from build123d import *
from OCP.BRepFilletAPI import BRepFilletAPI_MakeChamfer

# Parameters (mm, degrees)
BOSS_EXTRUDE1_DEPTH = 9
CUT_EXTRUDE1_REACH  = 32.118
SKETCH2_R           = 6.5
CUT_EXTRUDE2_DEPTH  = 18
CUT_EXTRUDE3_REACH  = 30.95
SKETCH4_R           = 3.7499999999999996
CUT_EXTRUDE4_DEPTH  = 10
FILLET1_R           = 2
CHAMFER1_SIZE       = 2
CHAMFER1_SIZE2      = 0.8842438837908889
CHAMFER1_SIZE2_2    = 0.8842438837908887


with BuildPart() as part:
    # Sketch1 → Boss-Extrude1 (new, symmetric)
    with BuildSketch(Plane.XY):
        Polygon((-25.633576548445145, 1e-17), (-11.506423451554879, 4e-17), (-8, 10), (0, 9.999999999999993), (8, 9.999999999999993), (11.506423451554879, 4e-17), (25.633576548445145, 4e-17), (25.63357654844514, 3.000000000000001), (13.633576548445141, 3), (10.12715309689026, 13.000000000000002), (0, 12.999999999999995), (-10.127153096890261, 13.000000000000002), (-13.633576548445141, 3), (-25.633576548445145, 3), align=None)
    extrude(amount=BOSS_EXTRUDE1_DEPTH, both=True)

    # Sketch2 → Cut-Extrude1 (cut, up to next)
    with BuildSketch(Plane(origin=(8.91e-15, 12.999999999999995, 0), x_dir=(1, -7.1e-16, 0), z_dir=(7.1e-16, 1, 0)), mode=Mode.PRIVATE) as cut_extrude1_sk1:
        with Locations(Location((0, 0, 0), (0, 0, 180))):
            Circle(SKETCH2_R)
    cut_extrude1_tool1 = extrude(cut_extrude1_sk1.sketch, amount=-CUT_EXTRUDE1_REACH, mode=Mode.PRIVATE) & part.part
    add(cut_extrude1_tool1.solids().sort_by_distance((0, 13, 0))[0], mode=Mode.SUBTRACT)

    # Sketch3 → Cut-Extrude2 (cut)
    with BuildSketch(Plane(origin=(8.91e-15, 12.999999999999995, 0), x_dir=(1, -7.1e-16, 0), z_dir=(7.1e-16, 1, 0))):
        Polygon((-10.12715309689027, 9), (-25.63357654844515, 4), (-25.63357654844515, 9), align=None)
        Polygon((-10.12715309689025, -9), (-25.63357654844515, -4), (-25.63357654844515, -9), align=None)
        Polygon((25.63357654844515, 9), (10.12715309689025, 9), (25.63357654844515, 4), align=None)
        Polygon((25.63357654844515, -4), (25.63357654844515, -9), (10.12715309689025, -9), align=None)
    extrude(amount=-CUT_EXTRUDE2_DEPTH, mode=Mode.SUBTRACT)

    # Sketch4 → Cut-Extrude3 (cut, up to next)
    with BuildSketch(Plane(origin=(0, 3, 0), x_dir=(1, 0, 0), z_dir=(0, 1, 0)), mode=Mode.PRIVATE) as cut_extrude3_sk1:
        with Locations(Location((-19.633576548445145, -2.4e-15, 0), (0, 0, 270))):
            Circle(SKETCH4_R)
    cut_extrude3_tool1 = extrude(cut_extrude3_sk1.sketch, amount=-CUT_EXTRUDE3_REACH, mode=Mode.PRIVATE) & part.part
    # Sketch4 → Cut-Extrude3 (cut, up to next)
    with BuildSketch(Plane(origin=(0, 3, 0), x_dir=(1, 0, 0), z_dir=(0, 1, 0)), mode=Mode.PRIVATE) as cut_extrude3_sk2:
        with Locations(Location((19.63357654844515, 2.4e-15, 0), (0, 0, 270))):
            Circle(SKETCH4_R)
    cut_extrude3_tool2 = extrude(cut_extrude3_sk2.sketch, amount=-CUT_EXTRUDE3_REACH, mode=Mode.PRIVATE) & part.part
    add(cut_extrude3_tool1.solids().sort_by_distance((-19.633577, 3, 0))[0], mode=Mode.SUBTRACT)
    add(cut_extrude3_tool2.solids().sort_by_distance((19.633577, 3, 0))[0], mode=Mode.SUBTRACT)

    # Sketch5 → Cut-Extrude4 (cut, symmetric)
    with BuildSketch(Plane.XY):
        Polygon((13.633576548445141, 3), (14.247200652467244, 1.2500000000000009), (25.63357654844515, 1.2500000000000009), (25.633576548445152, 3.000000000000001), align=None)
    extrude(amount=CUT_EXTRUDE4_DEPTH, both=True, mode=Mode.SUBTRACT)

    # Fillet1
    fillet1_edges = [part.edges().sort_by_distance(p)[0] for p in [
        (25.633576548445152, 0.6250000000000018, 4),
        (-25.633576548445145, 1.5, -4),
        (-25.633576548445145, 1.5, 4),
        (25.633576548445152, 0.6250000000000018, -4),
    ]]
    fillet(fillet1_edges, radius=FILLET1_R)

    # Chamfer1: one chamfer whose edges measure the first distance from different faces: ONE call of the kernel's chamfer builder (chamfer() names one face for all edges)
    chamfer1_edges_1 = [part.edges().sort_by_distance(p)[0] for p in [
        (14.247200652467244, 1.2500000000000009, 0),
    ]]
    chamfer1_side_1 = [part.faces().sort_by_distance(p)[0] for p in [
        (12.132458042687091, 7.281053120074241, 1.1e-16),
    ]]
    chamfer1_edges_2 = [part.edges().sort_by_distance(p)[0] for p in [
        (-13.633576548445141, 3, -3.55e-15),
    ]]
    chamfer1_side_2 = [part.faces().sort_by_distance(p)[0] for p in [
        (-11.841196306073245, 8.111705038297892, -3.84e-15),
    ]]
    chamfer1 = BRepFilletAPI_MakeChamfer(part.part.solid().wrapped)
    for e in chamfer1_edges_1:
        chamfer1.Add(CHAMFER1_SIZE, CHAMFER1_SIZE2, e.wrapped, chamfer1_side_1[0].wrapped)  # the first distance lies on this face
    for e in chamfer1_edges_2:
        chamfer1.Add(CHAMFER1_SIZE, CHAMFER1_SIZE2_2, e.wrapped, chamfer1_side_2[0].wrapped)  # the first distance lies on this face
    add(Compound.cast(chamfer1.Shape()), mode=Mode.REPLACE)


solid = part.part
Check sheet for the modelled part. Datum: model origin and axes. Units: mm. A direction names the side the tool comes from. Give positions to 0.01 mm unless a question says otherwise; leave off trailing zeros. Loops run counter-clockwise (first coordinate to the right, second up) from the corner with the lowest first, then second, coordinate; pieces in that order, holes last. Notation, with made-up numbers: M 35,-36.5 L 59,-36.5 A29 cw 59,-2.5 Z; hole C 84.25,-14 d11. An arc over 180 degrees is marked long. Answer as a JSON object with one key per item and string values. Group by question number.
Q1. Go/stop test with flat-tipped pins: P1, Ø5.5, axis at x = 23, z = -0.5, coming from the +Y side; P2, Ø4, axis at x = 16, z = -7, coming from the +Y side; P3, Ø1.5, axis at y = 10, z = 2.5, coming from the -X side. Record where each tip stops, or that it passes through.
Q2. Cross-section at A-A on z = 0. Record the cut outline in (x, y), then the cut area to 3 significant figures.
Q3. Cross-section at B-B on y = 2. Record the cut outline in (x, z), then the cut area to 3 significant figures.
Q4. Cross-section at C-C on x = 0. Record the cut outline in (y, z), then the cut area to 3 significant figures.
Q5. Release check for a two-part mould opening along Z. For faces 1 (the flat face through (15, 0, 0)), 2 (the cylindrical face through (-25.24, 1.479, 3.735)), 3 (the cylindrical face through (-23.294, 1.521, -0.813)) record: released by +Z, released by -Z, zero draft, split by the parting line, or undercut.
Q6. Cross-section at D-D on y = 6. Record the cut outline in (x, z).
Q7. Material ranges on line 1 along X through (y, z) = (0.8, 0); line 2 along X through (y, z) = (0.4, 0); line 3 along Y through (x, z) = (-6.5, 8), recorded low to high. Write a range as [from, to].
Q8. Access from +Z, -Z, +X, -X, +Y, -Y to the whole of each face (thin tool, end or side, straight path). Record for faces 4 (the cylindrical face through (25.24, 0.616, -3.735)), 5 (the cylindrical face through (-2.999, 11.521, -5.767)), 6 (the flat face through (-16, 3, 2)), 7 (the flat face through (9.73, 5.07, 0.13)), 8 (the flat face through (15.6, 1.25, 0.1)).
Evaluation:
{
 "1": {"P1": "stops at y = 1.25", "P2": "stops at y = 2.63", "P3": "stops at x = -11.44"},
 "2": {"outline": "M -25.63,0 L -23.38,0 L -23.38,3 L -25.63,3 Z; M -15.88,0 L -11.51,0 L -8,10 L -6.5,10 L -6.5,13 L -10.13,13 L -12.97,4.89 L -14.52,3 L -15.88,3 Z; M 6.5,10 L 8,10 L 11.51,0 L 15.88,0 L 15.88,1.25 L 15.13,1.25 L 13.59,3.14 L 10.13,13 L 6.5,13 Z; M 23.38,0 L 25.63,0 L 25.63,1.25 L 23.38,1.25 Z", "area": "107 mm2"},
 "3": {"outline": "M -25.63,-2.54 A2 ccw -24.25,-4.45 L -10.81,-8.78 L -10.81,8.78 L -24.25,4.45 A2 ccw -25.63,2.54 Z; M 10.81,-8.78 L 14.52,-7.58 L 14.52,7.58 L 10.81,8.78 Z; hole C -19.63,0 d7.5", "area": "205 mm2"},
 "4": {"outline": "M 10,-9 L 13,-9 L 13,-6.5 L 10,-6.5 Z; M 10,6.5 L 13,6.5 L 13,9 L 10,9 Z", "area": "15.0 mm2"},
 "5": {"face 1": "zero draft", "face 2": "released by +Z", "face 3": "undercut"},
 "6": {"outline": "M -12.58,-8.21 L -10.13,-9 L -9.4,-9 L -9.4,9 L -10.13,9 L -12.58,8.21 Z; M 9.4,-9 L 10.13,-9 L 12.58,-8.21 L 12.58,8.21 L 10.13,9 L 9.4,9 Z"},
 "7": {"line 1": "x = [-25.63, -23.38], [-15.88, -11.23], [11.23, 15.88], [23.38, 25.63]", "line 2": "x = [-25.63, -23.38], [-15.88, -11.37], [11.37, 15.88], [23.38, 25.63]", "line 3": "y = [10, 13]"},
 "8": {"face 4": "-Z, +X, +Y, -Y", "face 5": "+Y, -Y", "face 6": "+Z, -Z, -X, +Y", "face 7": "+Z, -Z, -Y", "face 8": "+Z, -Z, +X, +Y"}
}
